```python
from build123d import *

# Parameters (mm, degrees)
BOSS_EXTRUDE1_DEPTH     = 4
SKETCH2_R               = 1.5
SKETCH2_R_2             = 2.45
SKETCH2_R_3             = 1.499994387
SKETCH2_R_4             = 1.499990712
SKETCH2_W               = 22.5
SKETCH2_H               = 11.8
SKETCH2_W_2             = 3.2
SKETCH2_H_2             = 24.403689174
SKETCH2_W_3             = 3.200000004
CUT_EXTRUDE1_DEPTH      = 1
CUT_EXTRUDE1_DEPTH_BACK = 5
CUT_EXTRUDE2_DEPTH      = 1
CUT_EXTRUDE2_DEPTH_BACK = 5
FILLET1_R               = 10
FILLET2_R               = 5


with BuildPart() as part:
    # Sketch1 → Boss-Extrude1 (new body)
    with BuildSketch(Plane(origin=(0, 0, 0), x_dir=(1, 0, 0), z_dir=(0, 1, 0))):
        with BuildLine():
            Line((-120, 0), (-135, 0))
            ThreePointArc((-135, 0), (-138.535533906, -1.464466094), (-140, -5))
            Line((-140, -5), (-140, -20))
            Line((-140, -20), (-140, -160))
            ThreePointArc((-140, -160), (-134.142135624, -174.142135624), (-120, -180))
            Line((-120, -180), (-20, -180))
            ThreePointArc((-20, -180), (-5.857864376, -174.142135624), (0, -160))
            Line((0, -160), (0, -20))
            Line((0, -20), (0, -5))
            ThreePointArc((0, -5), (-1.464466094, -1.464466094), (-5, 0))
            Line((-5, 0), (-20, 0))
            Line((-20, 0), (-120, 0))
        make_face()
    extrude(amount=BOSS_EXTRUDE1_DEPTH)

    # Sketch2 → Cut-Extrude1 (cut, two sides)
    with BuildSketch(Plane(origin=(0, 4, 0), x_dir=(1, 0, 0), z_dir=(0, 1, 0))) as cut_extrude1_sk:
        with Locations((-80.3, -154.329714663)):
            Circle(SKETCH2_R)
        with Locations((-53, -154.329714663)):
            Circle(SKETCH2_R)
        with Locations((-6.5, -6.5)):
            Circle(SKETCH2_R_2)
        with Locations((-6.5, -48.5)):
            Circle(SKETCH2_R_2)
        with Locations((-133.5, -48.5)):
            Circle(SKETCH2_R_2)
        with Locations((-133.5, -6.5)):
            Circle(SKETCH2_R_2)
        with Locations((-82.507017072, -130.388178469)):
            Circle(SKETCH2_R_3)
        with Locations((-57.507017072, -130.388178469)):
            Circle(SKETCH2_R_4)
        with Locations((-76.676059564, -45.89557362)):
            Circle(SKETCH2_R)
        with Locations((-91.676059564, -45.89557362)):
            Circle(SKETCH2_R)
        with Locations((-76.676059564, -62.89557362)):
            Circle(SKETCH2_R)
        with Locations((-91.676059564, -62.89557362)):
            Circle(SKETCH2_R)
        with Locations((-94.5, -71.948209631)):
            Circle(SKETCH2_R)
        with Locations((-45.5, -71.948209631)):
            Circle(SKETCH2_R)
        with Locations((-94.5, -13.948209631)):
            Circle(SKETCH2_R)
        with Locations((-45.5, -13.948209631)):
            Circle(SKETCH2_R)
        with Locations((-126.081815918, -3.135397693)):
            Circle(SKETCH2_R)
        with Locations((-103.081815918, -3.135397693)):
            Circle(SKETCH2_R)
        with Locations((-126.081815918, -61.135397693)):
            Circle(SKETCH2_R)
        with Locations((-103.081815918, -61.135397693)):
            Circle(SKETCH2_R)
        with Locations((-130, -140.75)):
            Circle(SKETCH2_R)
        with Locations((-130, -154.25)):
            Circle(SKETCH2_R)
        with Locations((-10, -154.25)):
            Circle(SKETCH2_R)
        with Locations((-10, -140.75)):
            Circle(SKETCH2_R)
        with Locations((-66.65, -154.329714663)):
            Rectangle(SKETCH2_W, SKETCH2_H)
        with Locations((-91, -164.798155413)):
            Rectangle(SKETCH2_W_2, SKETCH2_H_2)
        with Locations((-46, -164.798155413)):
            Rectangle(SKETCH2_W_3, SKETCH2_H_2)
    extrude(amount=CUT_EXTRUDE1_DEPTH, mode=Mode.SUBTRACT)
    extrude(cut_extrude1_sk.sketch, amount=-CUT_EXTRUDE1_DEPTH_BACK, mode=Mode.SUBTRACT)

    # Sketch3 → Cut-Extrude2 (cut, two sides)
    with BuildSketch(Plane(origin=(0, 0, 0), x_dir=(-1, 0, 0), z_dir=(0, -1, 0))) as cut_extrude2_sk:
        with BuildLine():
            Line((0, -65), (28.307017072, -65))
            ThreePointArc((28.307017072, -65), (35.378084884, -67.928932188), (38.307017072, -75))
            Line((38.307017072, -75), (38.307017072, -115))
            ThreePointArc((38.307017072, -115), (35.378084884, -122.071067812), (28.307017072, -125))
            Line((28.307017072, -125), (0, -125))
            Line((0, -125), (0, -65))
        make_face()
        with BuildLine():
            Line((140, -65), (140, -125))
            Line((140, -125), (111.692982928, -125))
            ThreePointArc((111.692982928, -125), (104.621915116, -122.071067812), (101.692982928, -115))
            Line((101.692982928, -115), (101.692982928, -75))
            ThreePointArc((101.692982928, -75), (104.621915116, -67.928932188), (111.692982928, -65))
            Line((111.692982928, -65), (140, -65))
        make_face()
    extrude(amount=CUT_EXTRUDE2_DEPTH, mode=Mode.SUBTRACT)
    extrude(cut_extrude2_sk.sketch, amount=-CUT_EXTRUDE2_DEPTH_BACK, mode=Mode.SUBTRACT)

    # Fillet1
    fillet1_edges = [part.edges().sort_by_distance(p)[0] for p in [
        (0, 2, 125),
        (-140, 2, 125),
    ]]
    fillet(fillet1_edges, radius=FILLET1_R)

    # Fillet2
    fillet2_edges = [part.edges().sort_by_distance(p)[0] for p in [
        (0, 2, 65),
        (-140, 2, 65),
    ]]
    fillet(fillet2_edges, radius=FILLET2_R)


solid = part.part
```
The listing builds one solid part. Answer for the finished solid, in the listing's coordinates (mm). A direction names the side the tool comes from. Give positions to 0.01 mm unless a question says otherwise; leave off trailing zeros. Loops run counter-clockwise (first coordinate to the right, second up) from the corner with the lowest first, then second, coordinate; pieces in that order, holes last. Notation, with made-up numbers: (63.5, 72.25) - (67.5, 72.25) arc R17 ccw to (67.5, 81.25) - close; hole circle Ø4 at (5.25, 56.5). An arc over 180 degrees is marked (long way). Return JSON: item names as keys, results as strings. Group by question number.
1. Find section A-A (x = -24). Write down the section's boundary in (y, z).
2. Straight lines are drawn through the part: line 1 (Z direction, x = -94.5, y = 2.85); line 2 (X direction, y = 0.5, z = 161); line 3 (X direction, y = 3, z = 14). For each, find the intervals that lie inside material, in ascending order. Write a range as [from, to].
3. Determine the mould class of faces 1 (the flat face through (-67, 2, 160.23)), 2 (the cylindrical face through (-4.237, 2.028, 7.438)), 3 (the flat face through (-19, 2, 125)), 4 (the cylindrical face through (-2, 2, 64)) for opening direction X: pulls with the +X half, pulls with the -X half, needs draft (parallel to the pull), parting line crosses it, or undercut.
4. Which of the six approach directions +Z, -Z, +X, -X, +Y, -Y give full straight-line access (tool end or side, diameter ignored) to faces 5 (the flat face through (-38.307, 2, 95)), 6 (the flat face through (-101.693, 2, 95)), 7 (the flat face through (-89.4, 2, 165))?
5. Find section B-B (z = 109.5). Write down the section's boundary in (x, y).
6. Find section C-C (y = 3.4). State how many separate pieces and enclosed holes the cut face has, then the cut area to 3 significant figures.
7. Given pin 1 Ø1.2 at (y, z) = (2, 170.5) entering from -X; pin 2 Ø2 at (y, z) = (1.5, 161.5) entering from +X, each flat-ended and moving along its own axis, determine where each tip first touches the part or whether it passes through.
Verdict:
{
 "1": {"outline": "(0, 0) - (4, 0) - (4, 65) - (0, 65) - close; (0, 125) - (4, 125) - (4, 180) - (0, 180) - close"},
 "2": {"line 1": "z = [0, 12.45], [15.45, 70.45], [73.45, 180]", "line 2": "x = [-139.97, -92.6], [-89.4, -47.6], [-44.4, -0.03]", "line 3": "x = [-140, -96], [-93, -47], [-44, 0]"},
 "3": {"face 1": "undercut", "face 2": "undercut", "face 3": "needs draft", "face 4": "pulls with the +X half"},
 "4": {"face 5": "+X, +Y, -Y", "face 6": "-X, +Y, -Y", "face 7": "+Y, -Y"},
 "5": {"outline": "(-101.69, 0) - (-38.31, 0) - (-38.31, 4) - (-101.69, 4) - close"},
 "6": {"separate pieces": "1", "enclosed holes": "27", "area": "19,800 mm^2"},
 "7": {"pin 1": "stops at x = -137.38", "pin 2": "stops at x = -0.01"}
}
